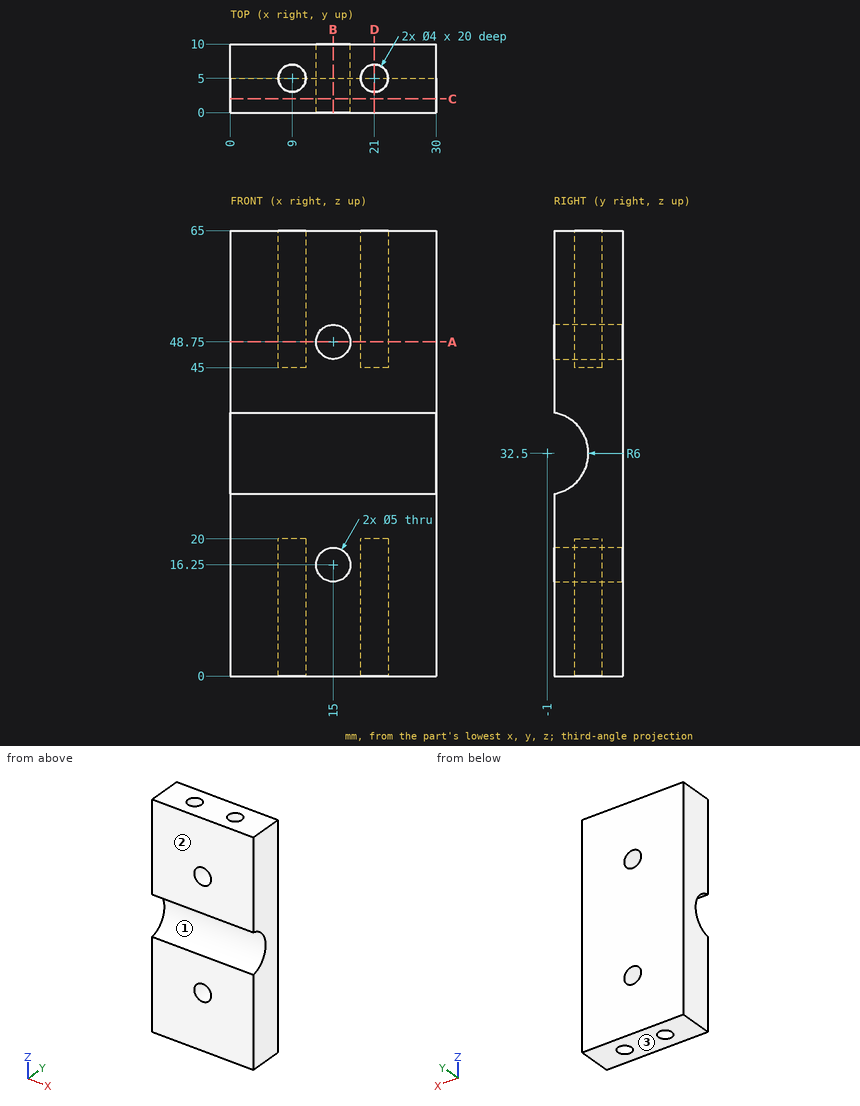
Can you work these out from the drawing? Everything is in mm from the part's minimum corner. Coordinates: 2 decimals unless noted, no trailing zeros. Write each loop counter-clockwise with the first axis right and the second up, starting at its lowest first coordinate (ties: lowest second). Pieces come first, ordered by that corner, then holes. Notation, with made-up numbers: (15, 83.25) - (41, 83.25) arc R12 ccw to (41, 98.25) - close; hole circle Ø5 at (57, 75.25). An arc over 180 degrees is marked (long way). One line per item, written item: value.
1) Suppose I cut it at D-D on x = 21. Write out the boundary of the cut face in (y, z).
Model answer:
outline: (0, 0) - (3, 0) - (3, 20) - (7, 20) - (7, 0) - (10, 0) - (10, 65) - (7, 65) - (7, 45) - (3, 45) - (3, 65) - (0, 65) - (0, 38.42) arc R6 cw to (0, 26.58) - close
2) We'd pull the mould along Z, two halves only. Please class the marked faces 1, 2 and 3: pulls with the +Z half, pulls with the -Z half, needs draft (parallel to the pull), parting line crosses it, or undercut.
Model answer:
face 1: undercut
face 2: needs draft
face 3: pulls with the -Z half
3) Suppose I cut it at A-A on z = 48.75. Write out the boundary of the cut face in (x, y), and give its area (3 significant figures).
Model answer:
outline: (0, 0) - (12.5, 0) - (12.5, 10) - (0, 10) - close; (17.5, 0) - (30, 0) - (30, 10) - (17.5, 10) - close; hole circle Ø4 at (9, 5); hole circle Ø4 at (21, 5)
area: 225 mm²
4) I'm going to push flat-ended pins straight in: P1, Ø3, axis at x = 9, y = 5, coming from the -Z side; P2, Ø3, axis at x = 15, z = 48.75, coming from the -Y side; P3, Ø1.2, axis at x = 21, y = 5.5, coming from the +Z side. Where does each tip first touch, or does it pass through?
Model answer:
P1: stops at z = 20
P2: passes through
P3: stops at z = 45
5) Suppose I cut it at B-B on x = 15. Write out the boundary of the cut face in (y, z), and give its area (3 significant figures).
Model answer:
outline: (0, 0) - (10, 0) - (10, 13.75) - (0, 13.75) - close; (0, 18.75) - (10, 18.75) - (10, 46.25) - (0, 46.25) - (0, 38.42) arc R6 cw to (0, 26.58) - close; (0, 51.25) - (10, 51.25) - (10, 65) - (0, 65) - close
area: 505 mm²
6) Suppose I cut it at C-C on y = 2. Write out the boundary of the cut face in (x, z).
Model answer:
outline: (0, 0) - (30, 0) - (30, 27.3) - (0, 27.3) - close; (0, 37.7) - (30, 37.7) - (30, 65) - (0, 65) - close; hole circle Ø5 at (15, 16.25); hole circle Ø5 at (15, 48.75)
7) I need wall thicknesses on line 1 along X through (y, z) = (2.75, 16.25); line 2 along Z through (x, y) = (16, 5.25); line 3 along Y through (x, z) = (21, 13.5). Which ranges of each line are inside material? Lowest first, please.
Model answer:
line 1: x = 0 to 12.5, 17.5 to 30
line 2: z = 0 to 13.96, 18.54 to 46.46, 51.04 to 65
line 3: y = 0 to 3, 7 to 10
